Verification items for the finished model (mm, model axes). A direction names the side the tool comes from. Give positions to 0.01 mm unless a question says otherwise; leave off trailing zeros. Order: outer loops, then holes, each group sorted by start corner. A loop starts at its lowest first (then second) coordinate and runs counter-clockwise, first axis right, second up.
(1) Scan lines: L1, parallel to Y at x = 101.5, z = 272.5; L2, parallel to X at y = -28.5, z = -264; L3, parallel to Y at x = 1, z = -355. Record each from-to range of solid material in increasing order.
(2) Sectioned sample at A-A on z = 117. Record the cut outline in (x, y).
(3) Sectioned sample at B-B on x = 112. Record the cut outline in (y, z).
(4) Access from +Z, -Z, +X, -X, +Y, -Y to the whole of each face (thin tool, end or side, straight path). Record for faces 1 (the face through (71, -1, -375)), 2 (the face through (1.5, -17, 5)).
(5) Gauge pin test, flat ends, axial feed: pin 1 (14.5 mm diameter, centred on y = -20, z = -145.5, fed in from +X); pin 2 (6 mm diameter, centred on x = 56, y = -4, fed in from -Z); pin 3 (12 mm diameter, centred on x = 101, z = -259.5, fed in from -Y). Record the tip position at first contact, or that the pin passes through.
```python
from build123d import *

# Parameters (mm, degrees)
SM_BASE_FLANGE_1_DEPTH = 375
SKETCH_7_R             = 3.5
CUT_EXTRUDE_1_DEPTH    = 10
CUT_EXTRUDE_2_DEPTH    = 10


# Sheet-metal steps are written as plain solids
with BuildPart() as part:
    # Sketch 1 → Базовая кромка1 (new, symmetric)
    with BuildSketch(Plane.XY):
        with BuildLine():
            Line((0, -32), (0, -3))
            ThreePointArc((0, -3), (0.878679656, -0.878679656), (3, 0))
            Line((3, 0), (141.5, 0))
            Line((141.5, 0), (141.5, -1.5))
            Line((141.5, -1.5), (3, -1.5))
            ThreePointArc((3, -1.5), (1.939339828, -1.939339828), (1.5, -3))
            Line((1.5, -3), (1.5, -32))
            Line((1.5, -32), (0, -32))
        make_face()
    extrude(amount=SM_BASE_FLANGE_1_DEPTH, both=True)

    # Эскиз7 → Вырез-Вытянуть1 (cut)
    with BuildSketch(Plane.ZY):
        with Locations((355, -19.5)):
            Circle(SKETCH_7_R)
    cut_extrude_1 = extrude(amount=-CUT_EXTRUDE_1_DEPTH, mode=Mode.SUBTRACT)

    # Эскиз8 → Вырез-Вытянуть2 (cut)
    with BuildSketch(Plane(origin=(0, 0, 0), x_dir=(1, 0, 0), z_dir=(0, 1, 0))):
        with BuildLine():
            Line((131.5, -328.5), (128.5, -328.5))
            ThreePointArc((128.5, -328.5), (125, -325), (128.5, -321.5))
            Line((128.5, -321.5), (131.5, -321.5))
            ThreePointArc((131.5, -321.5), (135, -325), (131.5, -328.5))
        make_face()
    cut_extrude_2 = extrude(amount=-CUT_EXTRUDE_2_DEPTH, mode=Mode.SUBTRACT)

    # Зеркальное отражение1: Вырез-Вытянуть1, Вырез-Вытянуть2 across plane
    add(cut_extrude_1.mirror(Plane.XY), mode=Mode.SUBTRACT)
    add(cut_extrude_2.mirror(Plane.XY), mode=Mode.SUBTRACT)


solid = part.part
```
Ans:
1. L1: y = -1.5 to 0
1. L2: x = 0 to 1.5
1. L3: y = -32 to -23, -16 to -0.76
2. outline: (0, -32) - (1.5, -32) - (1.5, -3) arc R1.5 cw to (3, -1.5) - (141.5, -1.5) - (141.5, 0) - (3, 0) arc R3 ccw to (0, -3) - close
3. outline: (-1.5, -375) - (0, -375) - (0, 375) - (-1.5, 375) - close
4. face 1: -Z, +X, -X, +Y, -Y
4. face 2: +Z, -Z, +X, -Y
5. pin 1: stops at x = 1.5
5. pin 2: stops at z = -375
5. pin 3: stops at y = -1.5
